```python
from build123d import *

# Parameters (mm, degrees)
SKETCH1_W           = 85
SKETCH1_H           = 95
BOSS_EXTRUDE1_DEPTH = 7
SKETCH2_W           = 30
SKETCH2_H           = 30
CUT_EXTRUDE1_DEPTH  = 7
SKETCH4_R           = 1.5
CUT_EXTRUDE2_DEPTH  = 10.5
SKETCH6_R           = 1.5
CUT_EXTRUDE3_DEPTH  = 8
CUT_EXTRUDE4_DEPTH  = 10
SKETCH8_R           = 1.5
CUT_EXTRUDE5_DEPTH  = 10
CUT_EXTRUDE6_DEPTH  = 5
SKETCH11_R          = 1.5
CUT_EXTRUDE8_DEPTH  = 4
SKETCH12_W          = 85
SKETCH12_H          = 7
CUT_EXTRUDE9_DEPTH  = 0.5


with BuildPart() as part:
    # Sketch1 → Boss-Extrude1 (new body)
    with BuildSketch(Plane.XY):
        with Locations((42.5, 47.5)):
            Rectangle(SKETCH1_W, SKETCH1_H)
    extrude(amount=BOSS_EXTRUDE1_DEPTH)

    # Sketch2 → Cut-Extrude1 (cut)
    with BuildSketch(Plane.XY.offset(7)):
        with Locations((42.5, 45)):
            Rectangle(SKETCH2_W, SKETCH2_H)
    extrude(amount=-CUT_EXTRUDE1_DEPTH, mode=Mode.SUBTRACT)

    # Sketch4 → Cut-Extrude2 (cut)
    with BuildSketch(Plane(origin=(0, 95, 0), x_dir=(1, 0, 0), z_dir=(0, 1, 0))):
        with Locations((21.25, -3.5)):
            Circle(SKETCH4_R)
        with Locations((63.75, -3.5)):
            Circle(SKETCH4_R)
    extrude(amount=-CUT_EXTRUDE2_DEPTH, mode=Mode.SUBTRACT)

    # Sketch6 → Cut-Extrude3 (cut)
    with BuildSketch(Plane(origin=(0, 0, 0), x_dir=(-1, 0, 0), z_dir=(0, 0, -1))):
        with Locations((-80.75, 90.75)):
            Circle(SKETCH6_R)
        with Locations((-4.25, 90.75)):
            Circle(SKETCH6_R)
        with Locations((-4.45, 4.25)):
            Circle(SKETCH6_R)
        with Locations((-80.75, 7.25)):
            Circle(SKETCH6_R)
    extrude(amount=-CUT_EXTRUDE3_DEPTH, mode=Mode.SUBTRACT)

    # Sketch7 → Cut-Extrude4 (cut)
    with BuildSketch(Plane(origin=(0, 0, 0), x_dir=(-1, 0, 0), z_dir=(0, 0, -1))):
        with BuildLine():
            Line((-85, 45), (-85, 0))
            Line((-85, 0), (0, 0))
            Line((0, 0), (0, 45))
            ThreePointArc((0, 45), (-42.5, 2.5), (-85, 45))
        make_face()
    extrude(amount=-CUT_EXTRUDE4_DEPTH, mode=Mode.SUBTRACT)

    # Sketch8 → Cut-Extrude5 (cut)
    with BuildSketch(Plane.XY.offset(7)):
        with Locations((80.75, 63)):
            Circle(SKETCH8_R)
        with Locations((4.25, 63)):
            Circle(SKETCH8_R)
    extrude(amount=-CUT_EXTRUDE5_DEPTH, mode=Mode.SUBTRACT)

    # Sketch9 → Cut-Extrude6 (cut)
    with BuildSketch(Plane(origin=(0, 0, 0), x_dir=(-1, 0, 0), z_dir=(0, 0, -1))):
        Polygon((-79.045, 65.953146627), (-82.455, 65.953146627), (-84.16, 63), (-82.455, 60.046853373), (-79.045, 60.046853373), (-77.34, 63), align=None)
        Polygon((-0.84, 63), (-2.545, 60.046853373), (-5.955, 60.046853373), (-7.66, 63), (-5.955, 65.953146627), (-2.545, 65.953146627), align=None)
    extrude(amount=-CUT_EXTRUDE6_DEPTH, mode=Mode.SUBTRACT)

    # Sketch11 → Cut-Extrude8 (cut)
    with BuildSketch(Plane.XY.offset(7)):
        with Locations((42.5, 6.75)):
            Circle(SKETCH11_R)
    extrude(amount=-CUT_EXTRUDE8_DEPTH, mode=Mode.SUBTRACT)

    # Sketch12 → Cut-Extrude9 (cut)
    with BuildSketch(Plane(origin=(0, 95, 0), x_dir=(1, 0, 0), z_dir=(0, 1, 0))):
        with Locations((42.5, -3.5)):
            Rectangle(SKETCH12_W, SKETCH12_H)
    extrude(amount=-CUT_EXTRUDE9_DEPTH, mode=Mode.SUBTRACT)


solid = part.part
```
For this review, take the finished solid that the model builds, in its own axes (mm). A direction names the side the tool comes from. Coordinates: 2 decimals unless noted, no trailing zeros. Order: outer loops, then holes, each group sorted by start corner. A loop starts at its lowest first (then second) coordinate and runs counter-clockwise, first axis right, second up. Notation, with made-up numbers: (-23, 55.5) -> (20, 55.5) arc R25 ccw to (20, 78.5) -> close; hole circle Ø6 at (45, -35.5). An arc over 180 degrees is marked (long way). Answer as CSV lines item,"result".
Q1. Draft analysis for pull direction Y (two halves, no side actions). For faces 6 (the face through (6.796, 61.503, 2.465)), 7 (the face through (65.18, 89.57, 3.05)), 8 (the face through (21, 84.5, 3)), state which applies: released by +Y, released by -Y, zero draft, split by the parting line, or undercut.
Model answer:
face 6,"undercut"
face 7,"zero draft"
face 8,"released by +Y"
Q2. Wall thickness on line 1 along X through (y, z) = (90.75, 3.75); line 2 along Y through (x, z) = (42.5, 5.5); line 3 along X through (y, z) = (90.5, 5.75): over which ranges is each line inside the solid? List them lowest first. Write a range as [from, to].
Model answer:
line 1,"x = [0, 2.75], [5.75, 19.77], [22.73, 62.27], [65.23, 79.25], [82.25, 85]"
line 2,"y = [2.5, 5.25], [8.25, 30], [60, 94.5]"
line 3,"x = [0, 2.77], [5.73, 79.27], [82.23, 85]"
Q3. We need section D-D (x = 21.25). State the section outline as (y, z) points.
Model answer:
outline,"(8.19, 0) -> (94.5, 0) -> (94.5, 2) -> (84.5, 2) -> (84.5, 5) -> (94.5, 5) -> (94.5, 7) -> (8.19, 7) -> close"
Q4. For faces 1 (the face through (42, 7, 3)), 2 (the face through (64, 84.5, 3)), 3 (the face through (27.5, 45, 4)), 4 (the face through (42, 70, 7)), 5 (the face through (1.704, 64.497, 2.465)), list the 3-axis set-ups (+Z, -Z, +X, -X, +Y, -Y) from which the entire face can be reached by the end or side of a thin tool; tool diameter is ignored.
Model answer:
face 1,"+Z"
face 2,"+Y"
face 3,"+Z, -Z"
face 4,"+Z, +X, -X, +Y, -Y"
face 5,"-Z"
Q5. Clearance check with flat-ended pins moving along their axes: pin 1 Ø3 at (x, y) = (5, 62.5) entering from -Z; pin 2 Ø1 at (y, z) = (23, 4.5) entering from +X; pin 3 Ø5 at (x, y) = (62, 70.5) entering from -Z; pin 4 Ø0.9 at (x, z) = (22, 3.5) entering from +Y. State where each tip first meets the part, or that it passes through.
Model answer:
pin 1,"stops at z = 5"
pin 2,"stops at x = 79.16"
pin 3,"stops at z = 0"
pin 4,"stops at y = 84.5"
Q6. We need section A-A (y = 90.75). State the section outline as (x, z) points.
Model answer:
outline,"(0, 0) -> (2.75, 0) -> (2.75, 7) -> (0, 7) -> close; (5.75, 0) -> (79.25, 0) -> (79.25, 7) -> (5.75, 7) -> close; (82.25, 0) -> (85, 0) -> (85, 7) -> (82.25, 7) -> close; hole circle Ø3 at (21.25, 3.5); hole circle Ø3 at (63.75, 3.5)"
Q7. We need section C-C (y = 51). State the section outline as (x, z) points, plus the area to 3 significant figures.
Model answer:
outline,"(0, 0) -> (27.5, 0) -> (27.5, 7) -> (0, 7) -> close; (57.5, 0) -> (85, 0) -> (85, 7) -> (57.5, 7) -> close"
area,"385 mm2"
Q8. We need section B-B (x = 50). State the section outline as (y, z) points.
Model answer:
outline,"(3.17, 0) -> (30, 0) -> (30, 7) -> (3.17, 7) -> close; (60, 0) -> (94.5, 0) -> (94.5, 7) -> (60, 7) -> close"
